Input: part model. Units: mm. Frame: model coordinates. Give positions to 0.01 mm unless a question says otherwise; leave off trailing zeros. Loops run counter-clockwise (first coordinate to the right, second up) from the corner with the lowest first, then second, coordinate; pieces in that order, holes last. Notation, with made-up numbers: (64.5, 60.25) -> (90.5, 60.25) arc R22 cw to (90.5, 95.25) -> close; hole circle Ø5 at (42, 7). An arc over 180 degrees is marked (long way). Answer in a Markdown table with one row per item. Add a question column.
Autodesk Inventor part; units mm, degrees
ref_plane "YZ Plane" through (0, 0, 0) normal (1, 0, 0) x (0, 1, 0)
ref_plane "XZ Plane" through (0, 0, 0) normal (0, 1, 0) x (-1, 0, 0)
ref_plane "XY Plane" through (0, 0, 0) normal (0, 0, 1) x (1, 0, 0)
ref_plane "Work Plane1" through (0, 0, 0) normal (0, 0, 1) x (1, 0, 0)
sketch "Sketch1" plane through (0, 0, 0) normal (0, 0, 1) x (1, 0, 0)
  line L0 (21.0929, -113.6856) -> (-23.9071, -113.6856)
  line L1 (-23.9071, -113.6856) -> (-23.9071, -103.6856)
  line L2 (-23.9071, -103.6856) -> (21.0929, -103.6856)
  line L3 (21.0929, -103.6856) -> (21.0929, -113.6856)
  line L4 (26.0929, -103.6856) -> (61.0929, -103.6856)
  line L5 (61.0929, -103.6856) -> (61.0929, -93.6856)
  line L6 (61.0929, -93.6856) -> (26.0929, -93.6856)
  line L7 (26.0929, -93.6856) -> (26.0929, -83.3195)
  line L8 (26.0929, -83.3195) -> (71.0929, -83.3195)
  line L9 (71.0929, -83.3195) -> (71.0929, -113.6856)
  line L10 (71.0929, -113.6856) -> (26.0929, -113.6856)
  line L11 (26.0929, -113.6856) -> (26.0929, -103.6856)
  line L12 (-13.9071, -83.6856) -> (21.0929, -83.6856)
  line L13 (21.0929, -83.6856) -> (21.0929, -93.6856)
  line L14 (21.0929, -93.6856) -> (-23.9071, -93.6856)
  line L15 (-23.9071, -93.6856) -> (-23.9071, -63.6856)
  line L16 (-23.9071, -63.6856) -> (21.0929, -63.6856)
  line L17 (21.0929, -63.6856) -> (21.0929, -73.6856)
  line L18 (21.0929, -73.6856) -> (-13.9071, -73.6856)
  line L19 (-13.9071, -73.6856) -> (-13.9071, -83.6856)
  line L20 (26.0929, -63.6856) -> (71.0929, -63.6856)
  line L21 (71.0929, -63.6856) -> (71.0929, -73.6856)
  line L22 (71.0929, -73.6856) -> (26.0929, -73.6856)
  line L23 (26.0929, -73.6856) -> (26.0929, -63.6856)
  line L24 (-28.9071, -63.6856) -> (-28.9071, -73.6856)
  line L25 (-28.9071, -73.6856) -> (-46.4071, -73.6856)
  line L26 (-46.4071, -73.6856) -> (-46.4071, -113.6856)
  line L27 (-46.4071, -113.6856) -> (-56.4071, -113.6856)
  line L28 (-56.4071, -113.6856) -> (-56.4071, -73.6856)
  line L29 (-56.4071, -73.6856) -> (-73.9071, -73.6856)
  line L30 (-73.9071, -73.6856) -> (-73.9071, -63.6856)
  line L31 (-73.9071, -63.6856) -> (-28.9071, -63.6856)
  line L32 (-103, 60.0133) -> (103, 60.0133)
  arc A0 (105, 58.0133) -> (103, 60.0133) centre (103, 58.0133) ccw
  line L33 (105, 58.0133) -> (105, 52.0133)
  arc A1 (103, 50.0133) -> (105, 52.0133) centre (103, 52.0133) ccw
  line L34 (103, 50.0133) -> (-103, 50.0133)
  arc A2 (-105, 52.0133) -> (-103, 50.0133) centre (-103, 52.0133) ccw
  line L35 (-105, 52.0133) -> (-105, 58.0133)
  arc A3 (-103, 60.0133) -> (-105, 58.0133) centre (-103, 58.0133) ccw
  line L36 (24.5, -38.5) -> (9.5, -38.5)
  line L37 (9.5, -38.5) -> (9.5, 36.5)
  line L38 (9.5, 36.5) -> (24.5, 36.5)
  line L39 (24.5, 36.5) -> (24.5, -38.5)
  line L40 (-110.5, 36.5) -> (-95.5, 36.5)
  line L41 (-95.5, 36.5) -> (-95.5, -38.5)
  line L42 (-95.5, -38.5) -> (-110.5, -38.5)
  line L43 (-110.5, -38.5) -> (-110.5, 36.5)
  line L44 (49.5, -38.5) -> (49.5, 36.5)
  line L45 (49.5, 36.5) -> (64.5, 36.5)
  line L46 (64.5, 36.5) -> (64.5, -38.5)
  line L47 (64.5, -38.5) -> (49.5, -38.5)
  line L48 (-15.5, -38.5) -> (-30.5, -38.5)
  line L49 (-30.5, -38.5) -> (-30.5, 36.5)
  line L50 (-30.5, 36.5) -> (-15.5, 36.5)
  line L51 (-15.5, 36.5) -> (-15.5, -38.5)
  line L52 (-55.5, 36.5) -> (-55.5, -38.5)
  line L53 (-55.5, -38.5) -> (-70.5, -38.5)
  line L54 (-70.5, -38.5) -> (-70.5, 36.5)
  line L55 (-70.5, 36.5) -> (-55.5, 36.5)
  line L56 (104.5, 36.5) -> (104.5, -38.5)
  line L57 (104.5, -38.5) -> (89.5, -38.5)
  line L58 (89.5, -38.5) -> (89.5, 36.5)
  line L59 (89.5, 36.5) -> (104.5, 36.5)
  circle A4 centre (29, 42) radius 2
  circle A5 centre (109, -56) radius 2
  circle A6 centre (-51, -56) radius 2
  circle A7 centre (-11, -56) radius 2
  circle A8 centre (-91, 42) radius 2
  circle A9 centre (69, 42) radius 2
  circle A10 centre (-11, 42) radius 2
  circle A11 centre (69, -56) radius 2
  circle A12 centre (-91, -56) radius 2
  circle A13 centre (29, -56) radius 2
  circle A14 centre (-51, 42) radius 2
  circle A15 centre (109, 42) radius 2
  line L60 (122.5, -135) -> (122.5, 75)
  line L61 (97.5, 75) -> (122.5, 75)
  line L62 (97.5, 70) -> (97.5, 75)
  line L63 (-97.5, 70) -> (97.5, 70)
  line L64 (-97.5, 70) -> (-97.5, 75)
  line L65 (-122.5, 75) -> (-97.5, 75)
  line L66 (-122.5, -135) -> (-122.5, 75)
  line L67 (-122.5, -135) -> (122.5, -135)
  point P0 (0, 0)
extrude "Plate1" add sketch "Sketch1" along normal blind 2
equation "\"d0\" = Thickness"
equation "\"BendRadius\" = Thickness"
equation "\"BendReliefWidth\" = Thickness"
equation "\"BendReliefDepth\" = 0.5 * Thickness"
equation "\"CornerReliefSize\" = 4 * Thickness"
equation "\"MinimumRemnant\" = 2 * Thickness"
equation "\"TransitionRadius\" = BendRadius"
equation "\"JacobiRadiusSize\" = BendRadius"
equation "\"GapSize\" = Thickness"
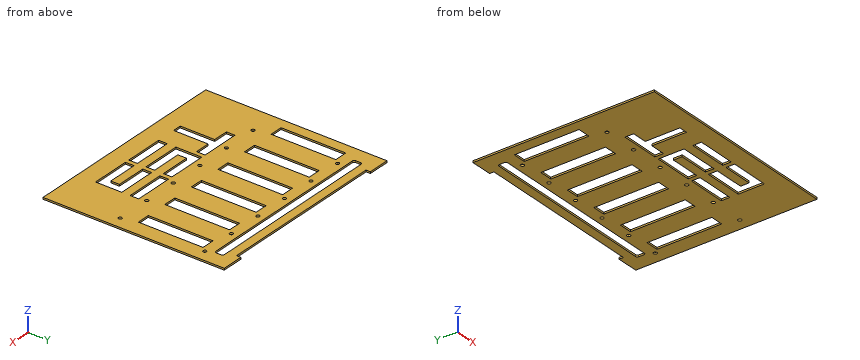
1) Section A-A on x = -85. Output: boundary loops of the cut face in (y, z), and give its area (3 significant figures).
2) Pin query (flat end, axial travel): pin 1 (0.6 mm diameter, centred on x = -49.5, z = 1.5, fed in from +Y). Return the tip coordinate at first contact, or that it passes through.
3) Section B-B on z = 1.5. State how many separate pieces and enclosed holes the cut face has, and give its area (3 significant figures).
4) Material intervals for line 1 along Y through (x, z) = (-46, 1.25); line 2 along Y through (x, z) = (-91, 1.1); line 3 along Y through (x, z) = (-24.5, 1.25), sorted ascending.
Working result:
| question | item | result |
|---|---|---|
| 1 | outline | (-135, 0) -> (50.01, 0) -> (50.01, 2) -> (-135, 2) -> close; (60.01, 0) -> (70, 0) -> (70, 2) -> (60.01, 2) -> close |
| 1 | area | 390 mm2 |
| 2 | pin 1 | stops at y = 70 |
| 3 | separate pieces | 1 |
| 3 | enclosed holes | 24 |
| 3 | area | 37,700 mm2 |
| 4 | line 1 | y = -135 to -73.69, -63.69 to 50.01, 60.01 to 70 |
| 4 | line 2 | y = -135 to -58, -54 to 40, 44 to 50.01, 60.01 to 70 |
| 4 | line 3 | y = -135 to -38.5, 36.5 to 50.01, 60.01 to 70 |
